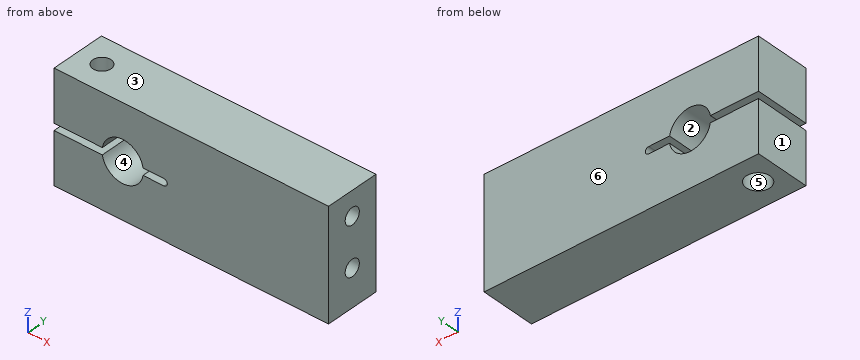
```python
from build123d import *

# Parameters (mm, degrees)
F0_W      = 63.5
F0_H      = 12.7
F1_DEPTH  = 25.4
F3_D      = 3.7973
F3_DEPTH  = 12.7
F3_TIP    = 1.1408240143
F4_D      = 3.7973
F4_DEPTH  = 12.7
F4_TIP    = 1.1408240143
F6_D      = 9.5504
F7_DEPTH  = 12.701
F10_D     = 5.5
F10_DEPTH = 11.9136
F12_D     = 4.2


with BuildPart() as f1:
    # F0 (on Top) → F1 (new body)
    with BuildSketch(Plane.XY):
        with Locations((-31.75, -6.35)):
            Rectangle(F0_W, F0_H)
    extrude(amount=F1_DEPTH)

    # F3
    with Locations(Plane.YZ):
        with Locations((-6.35, 19.812)):
            Hole(F3_D / 2, depth=F3_DEPTH)
            with Locations((0, 0, -(F3_DEPTH + F3_TIP / 2))):  # 118° drill point
                Cone(0, F3_D / 2, F3_TIP, mode=Mode.SUBTRACT)

    # F4
    with Locations(Plane.YZ):
        with Locations((-6.35, 8.636)):
            Hole(F4_D / 2, depth=F4_DEPTH)
            with Locations((0, 0, -(F4_DEPTH + F4_TIP / 2))):  # 118° drill point
                Cone(0, F4_D / 2, F4_TIP, mode=Mode.SUBTRACT)

    # F6 (through all)
    with Locations(Plane(origin=(0, 0, 0), x_dir=(-1, 0, 0), z_dir=(0, 1, 0))):
        with Locations((47.625, 12.7)):
            Hole(F6_D / 2)

    # F5 (on face) → F7 (cut, through all)
    with BuildSketch(Plane(origin=(0, 0, 0), x_dir=(-1, 0, 0), z_dir=(0, 1, 0))):
        with BuildLine():
            ThreePointArc((38.1, 13.4874), (37.3126, 12.7), (38.1, 11.9126))
            Line((38.1, 11.9126), (63.5, 11.9126))
            Line((63.5, 11.9126), (63.5, 12.7))
            Line((63.5, 12.7), (63.5, 13.4874))
            Line((63.5, 13.4874), (38.1, 13.4874))
        make_face()
    extrude(amount=-F7_DEPTH, mode=Mode.SUBTRACT)

    # F10 (through all, one way)
    with BuildSketch(Plane.XY.offset(11.9126)):
        with Locations((-57.9174169985, -6.35)):
            Circle(F10_D / 2)
    extrude(amount=-F10_DEPTH, mode=Mode.SUBTRACT)

    # F12 (through all)
    with Locations(Plane(origin=(0, 0, 13.4874), x_dir=(1, 0, 0), z_dir=(0, 0, -1))):
        with Locations((-57.8892030611, 6.35)):
            Hole(F12_D / 2)


solid = f1.part
```
Build history of the part. All positions in model axes, mm. Face numbers are marked on the shaded views. A direction names the side the tool comes from. Round coordinates to 2 decimals unless told otherwise and drop trailing zeros. Write each loop counter-clockwise with the first axis right and the second up, starting at its lowest first coordinate (ties: lowest second). Pieces come first, ordered by that corner, then holes. Notation, with made-up numbers: (32.25, 84) - (53.25, 84) arc R20 cw to (53.25, 106) - close; hole circle Ø10 at (65.25, 76). An arc over 180 degrees is marked (long way). Write each question's results on one line, items separated by ' | '. Start each with the question number.
Item 1: Saw through at C-C (x = -5). Write the cut outline in (y, z).
Item 2: Which spindle directions (+Z, -Z, +X, -X, +Y, -Y) get a long thin tool onto all of the face, cutting with end or side? Do the marked faces 4, 5 and 6. Say none if no direction does.
Item 3: Saw through at D-D (y = -7.25). State how many separate pieces and enclosed holes the cut face has, and give its area (3 significant figures).
Item 4: Saw through at B-B (y = -1.5). Write the cut outline in (x, z) (3 decimals), and give its area (3 significant figures).
Item 5: Saw through at A-A (z = 16.5). Write the cut outline in (x, y).
Item 6: Mould opens along Z. For the marked faces 1, 2 and 3 say: pulls with the +Z half, pulls with the -Z half, needs draft (parallel to the pull), parting line crosses it, or undercut.
Item 7: Drop flat-ended pins along their axis: P1, Ø5.5, axis at x = -57, y = -6.5, coming from the +Z side; P2, Ø2.5, axis at y = -6.35, z = 19.812, coming from the +X side. Give the stop position or say it passes through.
Item 8: Wall check: L1, parallel to Z at x = -5.5, y = -6.35; L2, parallel to Z at x = -38, y = -3.5; L3, parallel to X at y = -4.5, z = 15.75. Give the ranges that are in metal, low to high. Write a range as [from, to].
Results are:
1) outline: (-12.7, 0) - (0, 0) - (0, 25.4) - (-12.7, 25.4) - close; hole circle Ø3.8 at (-6.35, 8.64); hole circle Ø3.8 at (-6.35, 19.81)
2) face 4: +Y, -Y | face 5: -Z | face 6: +Z, -Z, +X, -X, +Y
3) separate pieces: 3 | enclosed holes: 0 | area: 1,320 mm²
4) outline: (-63.5, 0) - (0, 0) - (0, 25.4) - (-63.5, 25.4) - (-63.5, 13.487) - (-52.335, 13.487) arc R4.775 cw to (-42.915, 13.487) - (-38.1, 13.487) arc R0.787 cw to (-38.1, 11.913) - (-42.915, 11.913) arc R4.775 cw to (-52.335, 11.913) - (-63.5, 11.913) - close | area: 1,520 mm²
5) outline: (-63.5, -12.7) - (-50.52, -12.7) - (-50.52, 0) - (-63.5, 0) - close; (-44.73, -12.7) - (0, -12.7) - (0, 0) - (-44.73, 0) - close; hole circle Ø4.2 at (-57.89, -6.35)
6) face 1: needs draft | face 2: undercut | face 3: pulls with the +Z half
7) P1: stops at z = 25.4 | P2: stops at x = -13.09
8) L1: z = [0, 6.74], [10.53, 17.91], [21.71, 25.4] | L2: z = [0, 11.92], [13.48, 25.4] | L3: x = [-63.5, -58.88], [-56.9, -51.3], [-43.95, 0]
